Check sheet for the modelled part. Datum: model origin and axes. Units: mm. A direction names the side the tool comes from. Give positions to 0.01 mm unless a question says otherwise; leave off trailing zeros. Loops run counter-clockwise (first coordinate to the right, second up) from the corner with the lowest first, then second, coordinate; pieces in that order, holes last. Notation, with made-up numbers: (2.5, 31.25) -> (20.5, 31.25) arc R21 cw to (20.5, 69.25) -> close; hole circle Ø6 at (-12, -1). An arc over 180 degrees is marked (long way). Write each question's results on one line, items separated by ' | '. Start each with the question number.
Item 1: Access from +Z, -Z, +X, -X, +Y, -Y to the whole of each face (thin tool, end or side, straight path). Record for faces 4 (the face through (36.289, -295.405, 13.848)), 5 (the face through (9.392, -34.535, -40.974)).
Item 2: Cross-section at B-B on z = 5.5. Enter the section's corners in (x, y).
Item 3: Scan lines: line 1 along X through (y, z) = (-94, -4); line 2 along Y through (x, z) = (19, -48); line 3 along Y through (x, z) = (16, -32.5). Record each from-to range of solid material in increasing order.
Item 4: Cross-section at A-A on x = 15.5. Enter the section's corners in (y, z).
Item 5: Gauge pin test, flat ends, axial feed: pin 1 Ø3 at (x, y) = (33, -208.5) entering from -Z; pin 2 Ø12 at (y, z) = (-57.5, -24) entering from -X; pin 3 Ø4 at (x, y) = (7, -153) entering from -Z. Record the tip position at first contact, or that the pin passes through.
Item 6: Mould release check, pull along Y, two halves, no side actions. Record for faces 1 (the face through (38.1, -151, -28)), 2 (the face through (9.39, -126.66, -34.16)), 3 (the face through (1.91, -13.516, -0.635)): pulls with the +Y half, pulls with the -Y half, needs draft (parallel to the pull), parting line crosses it, or undercut.
from build123d import *

# Parameters (mm, degrees)
F1_DEPTH = 38.1
F3_DEPTH = 19.05
F4_R     = 6.35


with BuildPart() as f1:
    # F0 (on Right) → F1 (new body)
    with BuildSketch(Plane.YZ):
        Polygon((0, -89.2395835576), (0, 0), (-297.3143076455, 26.011631423), (-297.3143076455, 0.611631423), (-266.2792969737, -65.9431637408), align=None)
    extrude(amount=F1_DEPTH)

    # F2 (on face) → F3 (cut)
    with BuildSketch(Plane(origin=(0, 0, 0), x_dir=(0, -1, 0), z_dir=(-1, 0, 0))):
        Polygon((110.7021358254, 9.6851819128), (19.016308353, 1.663711403), (50.4944921991, -84.8218879197), (142.1803196716, -76.8004174098), align=None)
    extrude(amount=-F3_DEPTH, mode=Mode.SUBTRACT)

    # F4
    f4_edges = [f1.edges().sort_by_distance(p)[0] for p in [
        (0, -297.314308, 13.311631),
        (38.1, -297.314308, 13.311631),
        (38.1, -281.796802, -32.665766),
        (0, -281.796802, -32.665766),
        (19.05, -266.279297, -65.943164),
        (38.1, -133.139648, -77.591374),
        (38.1, 0, -44.619792),
        (19.05, 0, 0),
        (0, -25.247246, -87.030736),
        (0, -204.229808, -71.371791),
        (19.05, 0, -89.239584),
        (0, 0, -44.619792),
        (0, -9.508154, 0.831856),
        (19.05, -297.314308, 0.611631),
    ]]
    fillet(f4_edges, radius=F4_R)


solid = f1.part
Answer sheet:
1) face 4: +Z, -Z, +X, -Y | face 5: +Z, -X
2) outline: (0, -290.96) arc R6.35 ccw to (6.35, -297.31) -> (31.75, -297.31) arc R6.35 ccw to (38.1, -290.96) -> (38.1, -62.87) -> (19.05, -62.87) -> (19.05, -112.23) -> (0, -112.23) -> close
3) line 1: x = 19.05 to 38.1 | line 2: y = -274.65 to -131.7, -37.09 to 0 | line 3: y = -281.87 to -126.06, -31.45 to 0
4) outline: (-297.31, 2.02) arc R6.35 ccw to (-296.72, -0.66) -> (-267.83, -62.62) arc R6.35 ccw to (-262.63, -66.26) -> (-142.18, -76.8) -> (-110.7, 9.69) -> (-297.31, 26.01) -> close; (-50.49, -84.82) -> (-6.9, -88.64) arc R6.35 ccw to (0, -82.31) -> (0, -5.82) arc R6.35 ccw to (-5.8, 0.51) -> (-19.02, 1.66) -> close
5) pin 1: stops at z = -71.09 | pin 2: stops at x = 19.05 | pin 3: stops at z = -76.03
6) face 1: needs draft | face 2: undercut | face 3: pulls with the +Y half
